Read the model definition and answer for the solid it produces. Units are mm, in the model's axes. A direction names the side the tool comes from. Give positions to 0.01 mm unless a question says otherwise; leave off trailing zeros. Order: outer loops, then holes, each group sorted by start corner. A loop starts at its lowest first (then second) coordinate and runs counter-clockwise, first axis right, second up.
```python
from build123d import *

# Parameters (mm, degrees)
SKETCH_1_R          = 2.1
EXTRUDE_1_DEPTH     = 130
SKETCH_2_R          = 1.6
CUT_EXTRUDE_1_DEPTH = 10


with BuildPart() as part:
    # 草图1 → 凸台-拉伸1 (new body)
    with BuildSketch(Plane(origin=(0, 0, 0), x_dir=(1, 0, 0), z_dir=(0, 1, 0))):
        Polygon((5, 3.235022849), (-5, 3.235022849), (-5, 2.235022849), (-3.7, -0.016643201), (-3.7, -1.516643201), (-5, -3.76830925), (-5, -4.76830925), (5, -4.76830925), (5, -3.76830925), (3.7, -1.516643201), (3.7, -0.016643201), (5, 2.235022849), align=None)
        with Locations(Location((0, -0.766643201, 0), (0, 0, 270))):
            Circle(SKETCH_1_R, mode=Mode.SUBTRACT)
    extrude(amount=EXTRUDE_1_DEPTH)

    # 草图2 → 切除-拉伸1 (cut)
    with BuildSketch(Plane(origin=(0, 0, -3.235022849), x_dir=(-1, 0, 0), z_dir=(0, 0, -1))):
        with Locations((0, 126.8)):
            Circle(SKETCH_2_R)
        with Locations((0, 3.2)):
            Circle(SKETCH_2_R)
    extrude(amount=-CUT_EXTRUDE_1_DEPTH, mode=Mode.SUBTRACT)


solid = part.part
```
1) Consider L1, parallel to Y at x = 0, z = -2.05; L2, parallel to X at y = 126.8, z = 3.8; L3, parallel to Z at x = 0, y = 45. Determine where each line is inside the solid, lowest interval first.
Final values:
L1: y = 0 to 1.6, 4.8 to 125.2, 128.4 to 130
L2: x = -5 to -1.6, 1.6 to 5
L3: z = -3.24 to -1.33, 2.87 to 4.77
2) Given pin 1 (4 mm diameter, centred on x = -1, z = 2.5, fed in from -Y); pin 2 (1.6 mm diameter, centred on y = 50, z = 0.5, fed in from +X); pin 3 (1.2 mm diameter, centred on y = 79, z = 0.5, fed in from -X), each flat-ended and moving along its own axis, determine where each tip first touches the part or whether it passes through.
Final values:
pin 1: stops at y = 0
pin 2: stops at x = 3.88
pin 3: stops at x = -3.77
3) The part is cut by section C-C on y = 15.5. Determine the outline of the cut face in (x, z), and give its area (3 significant figures).
Final values:
outline: (-5, -3.24) - (5, -3.24) - (5, -2.24) - (3.7, 0.02) - (3.7, 1.52) - (5, 3.77) - (5, 4.77) - (-5, 4.77) - (-5, 3.77) - (-3.7, 1.52) - (-3.7, 0.02) - (-5, -2.24) - close; hole circle Ø4.2 at (0, 0.77)
area: 56.4 mm2
4) The part is cut by section A-A on x = 0. Determine the outline of the cut face in (y, z).
Final values:
outline: (0, -3.24) - (1.6, -3.24) - (1.6, -1.33) - (0, -1.33) - close; (0, 2.87) - (1.6, 2.87) - (1.6, 4.77) - (0, 4.77) - close; (4.8, -3.24) - (125.2, -3.24) - (125.2, -1.33) - (4.8, -1.33) - close; (4.8, 2.87) - (125.2, 2.87) - (125.2, 4.77) - (4.8, 4.77) - close; (128.4, -3.24) - (130, -3.24) - (130, -1.33) - (128.4, -1.33) - close; (128.4, 2.87) - (130, 2.87) - (130, 4.77) - (128.4, 4.77) - close
5) For a pull along Y with two mould halves and no side action, classify faces 1 (the face through (0, 64, -3.235)), 2 (the face through (-1.48, 2.59, -2.23)), 3 (the face through (-2.3, 130, 0.7)), 4 (the face through (-1.48, 126.19, -2.23)) as released by +Y, released by -Y, zero draft, split by the parting line, or undercut.
Final values:
face 1: zero draft
face 2: undercut
face 3: released by +Y
face 4: undercut
6) A tool of negligible diameter and unlimited length cuts with its end or side. For faces 5 (the face through (1.27, 2.23, 3.72)), 6 (the face through (-4.359, 64.09, -1.125)), 7 (the face through (4.36, 64.09, 2.66)), from which of +Z, -Z, +X, -X, +Y, -Y can it reach the whole face along a straight path? Write none if from no direction.
Final values:
face 5: +Z, -Z
face 6: -X, +Y, -Y
face 7: +X, +Y, -Y
7) The part is cut by section B-B on y = 126.8. Determine the outline of the cut face in (x, z), and give its area (3 significant figures).
Final values:
outline: (-5, -3.24) - (-1.6, -3.24) - (-1.6, -0.59) arc R2.1 cw to (-1.6, 2.13) - (-1.6, 4.77) - (-5, 4.77) - (-5, 3.77) - (-3.7, 1.52) - (-3.7, 0.02) - (-5, -2.24) - close; (1.6, -3.24) - (5, -3.24) - (5, -2.24) - (3.7, 0.02) - (3.7, 1.52) - (5, 3.77) - (5, 4.77) - (1.6, 4.77) - (1.6, 2.13) arc R2.1 cw to (1.6, -0.59) - close
area: 42.8 mm2
